CAD build for the part. Positions are in the model's coordinates, mm. Face numbers are marked on the shaded views. A direction names the side the tool comes from. Coordinates: 2 decimals unless noted, no trailing zeros. Loops run counter-clockwise (first coordinate to the right, second up) from the corner with the lowest first, then second, coordinate; pieces in that order, holes last. Notation, with made-up numbers: (25, -39.5) -> (61, -39.5) arc R22 cw to (61, -12.5) -> close; hole circle Ø3 at (66.25, -39). An arc over 180 degrees is marked (long way). Write each question's results on one line, items separated by ' | '.
```python
from build123d import *

# Parameters (mm, degrees)
SKETCH1_R           = 29
BOSS_EXTRUDE1_DEPTH = 55
SKETCH5_R           = 5
CUT_EXTRUDE2_DEPTH  = 45
SKETCH4_R           = 2.55
CUT_EXTRUDE1_DEPTH  = 69.607579756
CIRPATTERN2_COUNT   = 4
SKETCH6_R           = 12.5
CUT_EXTRUDE3_DEPTH  = 69.607579756
SKETCH8_R           = 3
CUT_EXTRUDE4_DEPTH  = 5
CUT_EXTRUDE5_DEPTH  = 1
CUT_EXTRUDE6_DEPTH  = 68.808554033
SKETCH12_R          = 3.9
CUT_EXTRUDE7_DEPTH  = 6
CUT_EXTRUDE8_DEPTH  = 45
SKETCH14_R          = 2.15
CUT_EXTRUDE9_DEPTH  = 69.607579756
SKETCH16_R          = 5.5
CUT_EXTRUDE10_DEPTH = 10


with BuildPart() as part:
    # Sketch1 → Boss-Extrude1 (new body)
    with BuildSketch(Plane(origin=(0, 0, 0), x_dir=(1, 0, 0), z_dir=(0, 1, 0))):
        with Locations(Location((0, 0, 0), (0, 0, 270))):
            Circle(SKETCH1_R)
    extrude(amount=BOSS_EXTRUDE1_DEPTH)

    # Sketch5 → Cut-Extrude2 (cut)
    with BuildSketch(Plane.XZ):
        with Locations(Location((-23, 0, 0), (0, 0, 270))):
            Circle(SKETCH5_R)
    cut_extrude2 = extrude(amount=-CUT_EXTRUDE2_DEPTH, mode=Mode.SUBTRACT)

    # Sketch4 → Cut-Extrude1 (cut, through all)
    with BuildSketch(Plane.XZ):
        with Locations(Location((-23, 0, 0), (0, 0, 270))):
            Circle(SKETCH4_R)
    cut_extrude1 = extrude(amount=-CUT_EXTRUDE1_DEPTH, mode=Mode.SUBTRACT)

    # CirPattern2: Cut-Extrude2, Cut-Extrude1 ×4 about axis
    cirpattern2_axis = Axis((0, 0, 0), (0, 1, 0))
    add([cut_extrude2.rotate(cirpattern2_axis, i * 360 / CIRPATTERN2_COUNT) for i in range(1, CIRPATTERN2_COUNT)], mode=Mode.SUBTRACT)
    add([cut_extrude1.rotate(cirpattern2_axis, i * 360 / CIRPATTERN2_COUNT) for i in range(1, CIRPATTERN2_COUNT)], mode=Mode.SUBTRACT)

    # Sketch6 → Cut-Extrude3 (cut, through all)
    with BuildSketch(Plane.XZ):
        with Locations(Location((0, 0, 0), (0, 0, 270))):
            Circle(SKETCH6_R)
    extrude(amount=-CUT_EXTRUDE3_DEPTH, mode=Mode.SUBTRACT)

    # Sketch8 → Cut-Extrude4 (cut)
    with BuildSketch(Plane.XZ):
        with Locations((-10.601366594, 26.239303084)):
            Circle(SKETCH8_R)
        with Locations((-26.239303084, -10.601366594)):
            Circle(SKETCH8_R)
        with Locations((10.601366594, -26.239303084)):
            Circle(SKETCH8_R)
        with Locations((26.239303084, 10.601366594)):
            Circle(SKETCH8_R)
    extrude(amount=-CUT_EXTRUDE4_DEPTH, mode=Mode.SUBTRACT)

    # Sketch9 → Cut-Extrude5 (cut)
    with BuildSketch(Plane.XZ):
        Polygon((20.610897481, -6.158537344), (22.597250544, -11.050653604), (12.998325456, -14.948119084), (11.011972394, -10.056002823), align=None)
    extrude(amount=-CUT_EXTRUDE5_DEPTH, mode=Mode.SUBTRACT)

    # Sketch11 → Cut-Extrude6 (cut, through all)
    with BuildSketch(Plane.XZ.offset(-1)):
        Polygon((22.102990836, -10.841856908), (20.402100785, -6.652797052), (11.506232102, -10.264799519), (13.207122153, -14.453859375), align=None)
    extrude(amount=-CUT_EXTRUDE6_DEPTH, mode=Mode.SUBTRACT)

    # Sketch12 → Cut-Extrude7 (cut)
    with BuildSketch(Plane.XZ):
        with Locations(Location((7.117525275, -17.616493237, 0), (0, 0, 270))):
            Circle(SKETCH12_R)
    extrude(amount=-CUT_EXTRUDE7_DEPTH, mode=Mode.SUBTRACT)

    # Sketch13 → Cut-Extrude8 (cut)
    with BuildSketch(Plane(origin=(0, 55, 0), x_dir=(1, 0, 0), z_dir=(0, 1, 0))):
        Polygon((18.745625864, -10.826118617), (20.450388629, -7.098234868), (18.074327983, -3.757925131), (13.993504571, -4.145499143), (12.288741806, -7.873382892), (14.664802452, -11.213692629), align=None)
        Polygon((-4.145499143, 13.993504571), (-3.757925131, 18.074327983), (-7.098234868, 20.450388629), (-10.826118617, 18.745625864), (-11.213692629, 14.664802452), (-7.873382892, 12.288741806), align=None)
        Polygon((-13.788869703, -16.687432566), (-9.829359199, -15.626484924), (-8.768411557, -11.666974419), (-11.666974419, -8.768411557), (-15.626484924, -9.829359199), (-16.687432566, -13.788869703), align=None)
    extrude(amount=-CUT_EXTRUDE8_DEPTH, mode=Mode.SUBTRACT)

    # Sketch14 → Cut-Extrude9 (cut, through all)
    with BuildSketch(Plane(origin=(0, 55, 0), x_dir=(1, 0, 0), z_dir=(0, 1, 0))):
        with Locations(Location((-7.48580888, 16.369565217, 0), (0, 0, 270))):
            Circle(SKETCH14_R)
        with Locations(Location((16.369565217, -7.48580888, 0), (0, 0, 270))):
            Circle(SKETCH14_R)
        with Locations(Location((-12.727922061, -12.727922061, 0), (0, 0, 270))):
            Circle(SKETCH14_R)
    extrude(amount=-CUT_EXTRUDE9_DEPTH, mode=Mode.SUBTRACT)

    # Sketch16 → Cut-Extrude10 (cut)
    with BuildSketch(Plane(origin=(0, 55, 0), x_dir=(1, 0, 0), z_dir=(0, 1, 0))):
        with Locations((0, 33)):
            Circle(SKETCH16_R)
        with Locations((0, -33)):
            Circle(SKETCH16_R)
    extrude(amount=-CUT_EXTRUDE10_DEPTH, mode=Mode.SUBTRACT)


solid = part.part
```
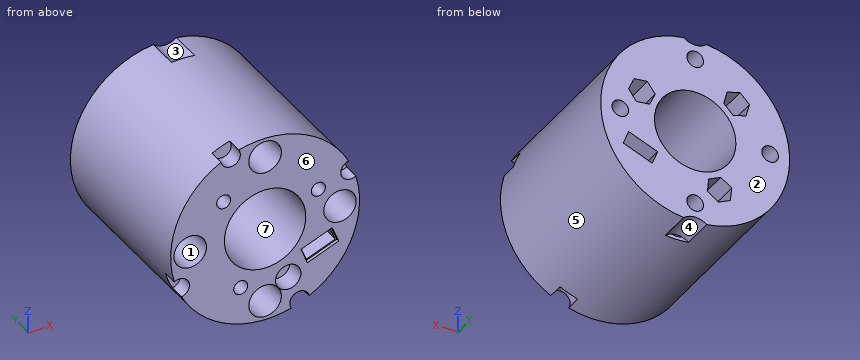
Q1. Wall check: L1, parallel to X at y = 43, z = 0; L2, parallel to X at y = 12, z = 7; L3, parallel to Z at x = -5.5, y = 34. Give the ranges that are in metal, low to high. Write a range as from..to.
Results are:
L1: -29..-28, -18..-12.5, 12.5..18, 28..29 | L2: -28.14..-10.36, 10.36..12.69, 20.38..28.14 | L3: -28.47..-19.31, -13.37..-11.22, 11.22..28.47
Q2. Cut at A-A on z = 0. Write the cut outline in (x, y).
Results are:
outline: (-29, 0) -> (-28, 0) -> (-28, 45) -> (-25.55, 45) -> (-25.55, 55) -> (-29, 55) -> close; (-20.45, 45) -> (-18, 45) -> (-18, 0) -> (-12.5, 0) -> (-12.5, 55) -> (-20.45, 55) -> close; (12.5, 0) -> (18, 0) -> (18, 45) -> (20.45, 45) -> (20.45, 55) -> (12.5, 55) -> close; (25.55, 45) -> (28, 45) -> (28, 0) -> (29, 0) -> (29, 55) -> (25.55, 55) -> close
Q3. Pull direction Z, two halves, no side cores. Call the marked faces 5, 6 and 7: +Z half, -Z half, draft (parallel to the pull), parting line (faces both ways), or undercut.
Results are:
face 5: parting line | face 6: draft | face 7: undercut
Q4. Which spindle directions (+Z, -Z, +X, -X, +Y, -Y) get a long thin tool onto all of the face, cutting with end or side? Do the marked faces 1, 2, 3 and 4. Say none if no direction does.
Results are:
face 1: -Y | face 2: +Z, -Z, +X, -X, +Y | face 3: +Z, +Y | face 4: -Z, +Y
Q5. Cut at C-C on y = 51. Give the number of separate pieces and of enclosed holes in the cut face, and give its area (3 significant figures).
Results are:
separate pieces: 1 | enclosed holes: 9 | area: 1,880 mm^2
Q6. Cut at B-B on x = 0. Write the cut outline in (y, z), and give its area (3 significant figures).
Results are:
outline: (0, -29) -> (45, -29) -> (45, -28) -> (0, -28) -> close; (0, -18) -> (45, -18) -> (45, -20.45) -> (55, -20.45) -> (55, -12.5) -> (0, -12.5) -> close; (0, 12.5) -> (55, 12.5) -> (55, 20.45) -> (45, 20.45) -> (45, 18) -> (0, 18) -> close; (0, 28) -> (45, 28) -> (45, 29) -> (0, 29) -> close; (45, -27.5) -> (55, -27.5) -> (55, -25.55) -> (45, -25.55) -> close; (45, 25.55) -> (55, 25.55) -> (55, 27.5) -> (45, 27.5) -> close | area: 783 mm^2
Q7. Drop flat-ended pins along their axis: pin 1 (6.5 mm diameter, centred on x = 23, z = 0, fed in from +Y); pin 2 (8 mm diameter, centred on x = -3, y = 8.5, fed in from -Z); pin 3 (3.5 mm diameter, centred on x = 10.5, z = -25.5, fed in from -Y); pin 4 (2.5 mm diameter, centred on x = 8, z = -19.5, fed in from -Y). Give the stop position or say it passes through.
Results are:
pin 1: y = 55 | pin 2: z = -29 | pin 3: y = 5 | pin 4: y = 6
